Check sheet for the modelled part. Datum: model origin and axes. Units: mm. Face numbers are marked on the shaded views. A direction names the side the tool comes from. Give positions to 0.01 mm unless a question says otherwise; leave off trailing zeros. Order: outer loops, then holes, each group sorted by start corner. A loop starts at its lowest first (then second) coordinate and runs counter-clockwise, first axis right, second up. Notation, with made-up numbers: (8, 71) -> (45, 71) arc R28 cw to (45, 104) -> close; hole circle Ø2 at (-18.75, 10.25). An arc over 180 degrees is marked (long way). Answer in a Markdown table with one row per item. Add a question column.
(1) Go/stop test with flat-tipped pins: pin 1 (6.5 mm diameter, centred on x = 1, z = 1.5, fed in from -Y); pin 2 (2 mm diameter, centred on x = 0, y = 14.5, fed in from -Z); pin 3 (10 mm diameter, centred on y = 17.5, z = 1, fed in from +X); pin 4 (5 mm diameter, centred on x = 0.5, y = 23, fed in from +Z). Record where each tip stops, or that it passes through.
(2) Cross-section at A-A (x = 0). Record the cut outline in (y, z), then the cut area to 3 significant figures.
(3) Set-up check for the marked faces 1, 2, 3, 4 and 5: record each of +Z, -Z, +X, -X, +Y, -Y from which the full face is reachable in a straight line by a thin tool's end or side.
(4) Thickness scan on L1, parallel to X at y = 14.5, z = 0; L2, parallel to X at y = 4, z = 0; L3, parallel to Y at x = 7.5, z = -6.5. Record the ranges inside material, lowest first. Write a range as [from, to].
(5) Release check for a two-part mould opening along Y. For the marked faces 6, 7, 8 and 9 record: released by +Y, released by -Y, zero draft, split by the parting line, or undercut.
(6) Cross-section at C-C (z = -8). Record the cut outline in (x, y), then the cut area to 3 significant figures.
(7) Cross-section at B-B (y = 18.5). Record the cut outline in (x, z), then the cut area to 3 significant figures.
(8) Cross-section at D-D (y = 4.5). Record the cut outline in (x, z), then the cut area to 3 significant figures.
```python
from build123d import *

# Parameters (mm, degrees)
SKETCH1_R              = 10
SKETCH1_R_2            = 4
BOSS_EXTRUDE1_DEPTH    = 9
BOSS_EXTRUDE2_DEPTH    = 20
SKETCH5_R              = 4
CUT_EXTRUDE3_DEPTH     = 13
FILLET1_R              = 3
M4_TAPPED_HOLE1_REACH  = 35.17
M4_TAPPED_HOLE1_BORE_R = 1.65
CIRPATTERN1_COUNT      = 2
CIRPATTERN1_ANGLE      = 120


with BuildPart() as part:
    # Sketch1 → Boss-Extrude1 (new body)
    with BuildSketch(Plane(origin=(0, 0, 0), x_dir=(1, 0, 0), z_dir=(0, 1, 0))):
        with Locations(Location((0, 0, 0), (0, 0, 270))):
            Circle(SKETCH1_R)
        with Locations(Location((0, 0, 0), (0, 0, 270))):
            Circle(SKETCH1_R_2, mode=Mode.SUBTRACT)
    extrude(amount=BOSS_EXTRUDE1_DEPTH)

    # Sketch4 → Boss-Extrude2 (add)
    with BuildSketch(Plane(origin=(0, 9, 0), x_dir=(1, 0, 0), z_dir=(0, 1, 0))):
        with BuildLine():
            Line((-3.31662479, -5), (3.31662479, -5))
            ThreePointArc((3.31662479, -5), (6, 0), (3.31662479, 5))
            Line((3.31662479, 5), (-3.31662479, 5))
            ThreePointArc((-3.31662479, 5), (-6, 0), (-3.31662479, -5))
        make_face()
    extrude(amount=BOSS_EXTRUDE2_DEPTH)

    # Sketch5 → Cut-Extrude3 (cut)
    with BuildSketch(Plane.XZ.offset(-9)):
        with Locations(Location((0, 0, 0), (0, 0, 270))):
            Circle(SKETCH5_R)
    extrude(amount=-CUT_EXTRUDE3_DEPTH, mode=Mode.SUBTRACT)

    # Fillet1
    fillet1_edges = [part.edges().sort_by_distance(p)[0] for p in [
        (3.31662479, 19, 5),
        (3.31662479, 19, -5),
        (-3.31662479, 19, -5),
        (-3.31662479, 19, 5),
    ]]
    fillet(fillet1_edges, radius=FILLET1_R)

    # M4 Tapped Hole1 bore (on position points) → M4 Tapped Hole1 (cut, up to next)
    with BuildSketch(Plane(origin=(0, 4.5, -10), x_dir=(-1, 0, 0), z_dir=(0, 0, -1)), mode=Mode.PRIVATE) as m4_tapped_hole1_sk1:
        Circle(M4_TAPPED_HOLE1_BORE_R)
    m4_tapped_hole1_tool1 = extrude(m4_tapped_hole1_sk1.sketch, amount=-M4_TAPPED_HOLE1_REACH, mode=Mode.PRIVATE) & part.part
    m4_tapped_hole1 = m4_tapped_hole1_tool1.solids().sort_by_distance((0, 4.5, -10))[0]
    add(m4_tapped_hole1, mode=Mode.SUBTRACT)

    # CirPattern1: M4 Tapped Hole1 ×2 about axis
    cirpattern1_axis = Axis((0, 9, 0), (0, 1, 0))
    for i in range(1, CIRPATTERN1_COUNT):
        add(m4_tapped_hole1.rotate(cirpattern1_axis, i * CIRPATTERN1_ANGLE / (CIRPATTERN1_COUNT - 1)), mode=Mode.SUBTRACT)


solid = part.part
```
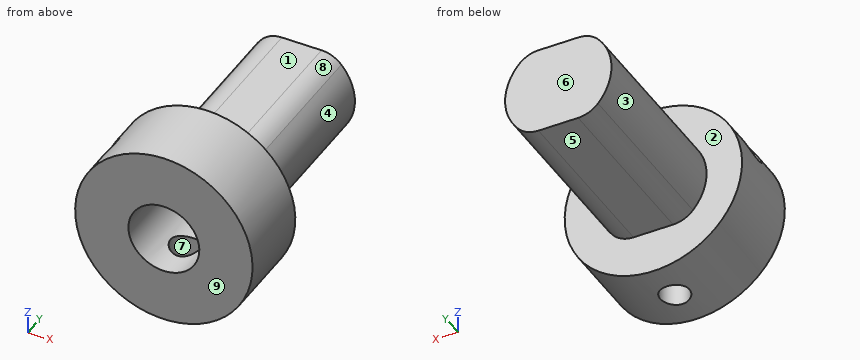
Answer below:
| question | item | result |
|---|---|---|
| 1 | pin 1 | stops at y = 0 |
| 1 | pin 2 | stops at z = -5 |
| 1 | pin 3 | stops at x = 6 |
| 1 | pin 4 | stops at z = 5 |
| 2 | outline | (0, -10) -> (2.85, -10) -> (2.85, -4) -> (0, -4) -> close; (0, 4) -> (22, 4) -> (22, -4) -> (6.15, -4) -> (6.15, -10) -> (9, -10) -> (9, -5) -> (29, -5) -> (29, 5) -> (9, 5) -> (9, 10) -> (0, 10) -> close |
| 2 | area | 184 mm² |
| 3 | face 1 | +Z, +X, -X, +Y |
| 3 | face 2 | +Y |
| 3 | face 3 | -X, +Y |
| 3 | face 4 | +X, +Y |
| 3 | face 5 | -Z, +X, -X, +Y |
| 4 | L1 | x = [-6, -4], [4, 6] |
| 4 | L2 | x = [-10, -4], [4, 10] |
| 4 | L3 | y = [0, 9] |
| 5 | face 6 | released by +Y |
| 5 | face 7 | undercut |
| 5 | face 8 | zero draft |
| 5 | face 9 | released by -Y |
| 6 | outline | (-6, 0) -> (6, 0) -> (6, 9) -> (-6, 9) -> close; hole circle Ø3.3 at (0, 4.5) |
| 6 | area | 99.4 mm² |
| 7 | outline | (-4.47, -4) arc R3 ccw to (-2.24, -5) -> (2.24, -5) arc R3 ccw to (4.47, -4) arc R6 ccw to (4.47, 4) arc R3 ccw to (2.24, 5) -> (-2.24, 5) arc R3 ccw to (-4.47, 4) arc R6 ccw to start; hole circle Ø8 at (0, 0) |
| 7 | area | 53.2 mm² |
| 8 | outline | (-9.37, 3.5) arc R10 ccw to (-1.65, -9.86) -> (-1.65, -3.64) arc R4 cw to (-3.98, 0.39) -> close; (-7.72, 6.36) -> (-2.33, 3.25) arc R4 cw (long way) to (1.65, -3.64) -> (1.65, -9.86) arc R10 ccw (long way) to start |
| 8 | area | 224 mm² |
